Work out the finished part from the listing and answer in its coordinate system (mm). Coordinates: 2 decimals unless noted, no trailing zeros. Order: outer loops, then holes, each group sorted by start corner. A loop starts at its lowest first (then second) coordinate and runs counter-clockwise, first axis right, second up.
1. The part is cut by section B-B, the plane z = 21. Give the vertices of the cut face in (x, y), then the cut area to 3 significant figures.
2. The part is cut by section A-A, the plane y = 31.5. Give the vertices of the cut face in (x, z).
3. The part is cut by section D-D, the plane z = 34.5. Give the vertices of the cut face in (x, y), then the cut area to 3 significant figures.
4. The part is cut by section C-C, the plane y = 8. Give the vertices of the cut face in (x, z).
5. Flat-ended cylindrical pins translate along their axes: pin 1 Ø0.5 at (x, z) = (1.5, 19) entering from -Y; pin 2 Ø0.9 at (x, y) = (1.5, 30.5) entering from +Z; pin 3 Ø1 at (x, z) = (1.5, 20.5) entering from -Y. Find the tip coordinate at first contact, or state that the pin passes through.
6. Find the intervals of material crossed by probe 1 along Y at (x, z) = (1.85, 22); probe 2 along Z at (x, y) = (2.2, 31.5); probe 3 along Z at (x, y) = (2.3, 4), in increasing order.
```python
from build123d import *

# Parameters (mm, degrees)
F1_DEPTH = 3


with BuildPart() as f1:
    # F0 (on Right) → F1 (new body)
    with BuildSketch(Plane.YZ):
        Polygon((20.5, 0), (24, 0), (24, 3), (34, 3), (34, 0), (41, 0), (41, 7), (44, 7), (44, 17), (41, 17), (41, 19.5), (34.5, 19.5), (34.5, 18.5), (32.5, 18.5), (32.5, 19.5), (29, 19.5), (29, 20.5), (29, 21.5), (32.5, 21.5), (32.5, 22.5), (34.5, 22.5), (34.5, 21.5), (41, 21.5), (41, 24), (44, 24), (44, 34), (41, 34), (41, 41), (34, 41), (34, 38), (24, 38), (24, 41), (20.5, 41), (17, 41), (17, 38), (7, 38), (7, 41), (0, 41), (0, 34), (-3, 34), (-3, 24), (0, 24), (0, 21.5), (6.5, 21.5), (6.5, 22.5), (8.5, 22.5), (8.5, 21.5), (12, 21.5), (12, 20.5), (12, 19.5), (8.5, 19.5), (8.5, 18.5), (6.5, 18.5), (6.5, 19.5), (0, 19.5), (0, 17), (-3, 17), (-3, 7), (0, 7), (0, 0), (7, 0), (7, 3), (17, 3), (17, 0), align=None)
    extrude(amount=F1_DEPTH)


solid = f1.part
```
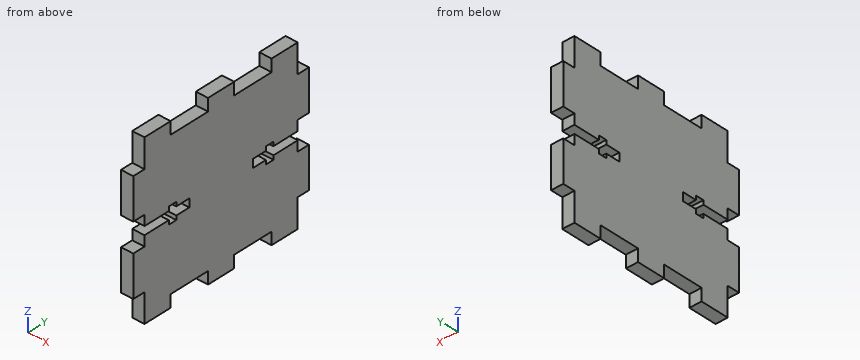
Geometry says:
1. outline: (0, 12) - (3, 12) - (3, 29) - (0, 29) - close
1. area: 51.0 mm2
2. outline: (0, 3) - (3, 3) - (3, 19.5) - (0, 19.5) - close; (0, 21.5) - (3, 21.5) - (3, 38) - (0, 38) - close
3. outline: (0, 0) - (3, 0) - (3, 41) - (0, 41) - close
3. area: 123 mm2
4. outline: (0, 3) - (3, 3) - (3, 18.5) - (0, 18.5) - close; (0, 22.5) - (3, 22.5) - (3, 38) - (0, 38) - close
5. pin 1: stops at y = 0
5. pin 2: stops at z = 38
5. pin 3: stops at y = 12
6. probe 1: y = 0 to 6.5, 8.5 to 32.5, 34.5 to 41
6. probe 2: z = 3 to 19.5, 21.5 to 38
6. probe 3: z = 0 to 19.5, 21.5 to 41
